from build123d import *

# Parameters (mm, degrees)
EXTRUDE_1_DEPTH = 10


with BuildPart() as part:
    # Эскиз1 → Вытянуть1 (new body)
    with BuildSketch(Plane(origin=(0, 0, 0), x_dir=(0, 0, -1), z_dir=(1, 0, 0))):
        with BuildLine():
            Line((26.672393858, 176.18957543), (35.064656469, 209.758625876))
            ThreePointArc((35.064656469, 209.758625876), (34.509070686, 212.952387038), (31.769638193, 214.68567742))
            ThreePointArc((31.769638193, 214.68567742), (0, 217.023616226), (-31.769638193, 214.68567742))
            ThreePointArc((-31.769638193, 214.68567742), (-34.509070686, 212.952387038), (-35.064656469, 209.758625876))
            Line((-35.064656469, 209.758625876), (-26.672393858, 176.18957543))
            ThreePointArc((-26.672393858, 176.18957543), (-25.418843537, 174.143301579), (-23.219791878, 173.182678407))
            ThreePointArc((-23.219791878, 173.182678407), (0, 171.936937008), (23.219791878, 173.182678407))
            ThreePointArc((23.219791878, 173.182678407), (25.418843537, 174.143301579), (26.672393858, 176.18957543))
        make_face()
        with BuildLine():
            Line((13.715292518, 182.861170071), (18.86026165, 203.441046598))
            ThreePointArc((18.86026165, 203.441046598), (18.220421187, 206.755900608), (15.272036319, 208.400491618))
            ThreePointArc((15.272036319, 208.400491618), (0, 208.959326186), (-15.272036319, 208.400491618))
            ThreePointArc((-15.272036319, 208.400491618), (-18.220421187, 206.755900608), (-18.86026165, 203.441046598))
            Line((-18.86026165, 203.441046598), (-13.715292518, 182.861170071))
            ThreePointArc((-13.715292518, 182.861170071), (-12.371326308, 180.738475491), (-10.026657624, 179.835920111))
            ThreePointArc((-10.026657624, 179.835920111), (0, 179.595223033), (10.026657624, 179.835920111))
            ThreePointArc((10.026657624, 179.835920111), (12.371326308, 180.738475491), (13.715292518, 182.861170071))
        make_face(mode=Mode.SUBTRACT)
    extrude(amount=EXTRUDE_1_DEPTH)


solid = part.part
Could you check a few things on this model? Use its own coordinates, in mm. A direction names the side the tool comes from. Round coordinates to 2 decimals unless told otherwise and drop trailing zeros. Order: outer loops, then holes, each group sorted by start corner. A loop starts at its lowest first (then second) coordinate and runs counter-clockwise, first axis right, second up.
(1) Please list where these lines run through material, in increasing order: line 1 along Y through (x, z) = (4.5, -2); line 2 along Y through (x, z) = (4.5, 1); line 3 along Z through (x, y) = (0.75, 198.5) (3 decimals).
Response values:
line 1: y = 171.95 to 179.6, 208.95 to 217.01
line 2: y = 171.94 to 179.6, 208.96 to 217.02
line 3: z = -32.25 to -17.625, 17.625 to 32.25
(2) Imagine slicing it at C-C (y = 198). Write out the boundary of the cut face in (x, z) (3 decimals), plus the area to 4 significant figures.
Response values:
outline: (0, -32.125) - (10, -32.125) - (10, -17.5) - (0, -17.5) - close; (0, 17.5) - (10, 17.5) - (10, 32.125) - (0, 32.125) - close
area: 292.5 mm2
(3) Imagine slicing it at B-B (z = -6). Write out the boundary of the cut face in (x, y).
Response values:
outline: (0, 172.02) - (10, 172.02) - (10, 179.68) - (0, 179.68) - close; (0, 208.87) - (10, 208.87) - (10, 216.94) - (0, 216.94) - close
(4) Which directions (+Z, -Z, +X, -X, +Y, -Y) give clear straight access to the entire face, cutting with the end or side of a thin tool? Please do faces 5 (the cylindrical face through (4.93, 171.937, 0.326)), 6 (the flat face through (4.93, 193.295, 16.324)).
Response values:
face 5: +X, -X, -Y
face 6: +X, -X
(5) If we mould it in two halves opening along Y, with no side actions, what happens to faces 1 (the cylindrical face through (4.93, 180.716, -12.344)), 2 (the cylindrical face through (4.93, 217.023, -0.446)), 3 (the flat face through (4.9, 192.7, -30.8)), 4 (the flat face through (0, 210, 0))? For each: released by +Y, released by -Y, zero draft, split by the parting line, or undercut.
Response values:
face 1: undercut
face 2: released by +Y
face 3: released by -Y
face 4: zero draft
(6) Imagine slicing it at D-D (y = 175.5). Write out the boundary of the cut face in (x, z), plus the area to 3 significant figures.
Response values:
outline: (0, -26.43) - (10, -26.43) - (10, 26.43) - (0, 26.43) - close
area: 529 mm2
(7) I'm going to push flat-ended pins straight in: pin 1 (5 mm diameter, centred on x = 9, z = -7, fed in from +Y); pin 2 (3 mm diameter, centred on x = 8, y = 198, fed in from -Z); pin 3 (3 mm diameter, centred on x = 4.5, y = 207.5, fed in from +Z) (3 decimals); pin 4 (5 mm diameter, centred on y = 203, z = 15.5, fed in from +X). Where does each tip first touch, or does it pass through?
Response values:
pin 1: stops at y = 216.98
pin 2: stops at z = -32.5
pin 3: stops at z = 34.875
pin 4: passes through
(8) Imagine slicing it at A-A (x = 6.5). Write out the boundary of the cut face in (y, z), plus the area to 3 significant figures.
Response values:
outline: (173.18, -23.22) arc R4 ccw to (176.19, -26.67) - (209.76, -35.06) arc R4 ccw to (214.69, -31.77) arc R217.02 ccw to (214.69, 31.77) arc R4 ccw to (209.76, 35.06) - (176.19, 26.67) arc R4 ccw to (173.18, 23.22) arc R217.02 ccw to start; hole (179.84, -10.03) arc R4 ccw to (182.86, -13.72) - (203.44, -18.86) arc R4 ccw to (208.4, -15.27) arc R208.96 ccw to (208.4, 15.27) arc R4 ccw to (203.44, 18.86) - (182.86, 13.72) arc R4 ccw to (179.84, 10.03) arc R208.96 ccw to start
area: 1,760 mm2
